```python
from build123d import *

# Parameters (mm, degrees)
EXTRUDE004_DEPTH                     = 120
EXTRUDE004_ONTO_SKETCH004_ROLL_ANGLE = 90
ARRAY005_X_COUNT                     = 2
ARRAY005_X_PITCH                     = 51
EXTRUDE001_DEPTH                     = 120
EXTRUDE001_ONTO_SKETCH001_ROLL_ANGLE = 90
ARRAY003_Z_COUNT                     = 2
ARRAY003_Z_PITCH                     = 21
BOX001_W                             = 96
BOX001_H                             = 118
BOX001_DEPTH                         = 41
BOX_W                                = 102
BOX_H                                = 120
BOX_DEPTH                            = 47
FILLET_R                             = 0.5
EXTRUDE003_DEPTH                     = 119
EXTRUDE003_ONTO_SKETCH003_ROLL_ANGLE = 90
ARRAY_X_COUNT                        = 2
ARRAY_X_PITCH                        = 51
EXTRUDE002_DEPTH                     = 119
EXTRUDE002_ONTO_SKETCH002_ROLL_ANGLE = 90
ARRAY004_Z_COUNT                     = 2
ARRAY004_Z_PITCH                     = 21
EXTRUDE_DEPTH                        = 0.8
ARRAY002_X_COUNT                     = 8
ARRAY002_X_PITCH                     = 12


with BuildPart() as bottomsideguidearray:
    # Sketch004 as drawn → Extrude004 (new)
    with BuildSketch(Plane.XY):
        Polygon((-6, 1), (4, 1), (2, -1), (-4, -1), align=None)
    extrude(amount=-EXTRUDE004_DEPTH)


with BuildPart() as bottomsideguidearray_1:
    # Extrude004 onto Sketch004 roll: moved
    add(bottomsideguidearray.part.rotate(Axis((0, 0, 0), (1, 0, 0)), EXTRUDE004_ONTO_SKETCH004_ROLL_ANGLE))


with BuildPart() as bottomsideguidearray_2:
    # Extrude004 onto Sketch004 placement: moved
    add(bottomsideguidearray_1.part)


with BuildPart() as bottomsideguidearray_3:
    # Extrude004 placement: moved
    add(bottomsideguidearray_2.part.moved(Location((25.5, 0, 0))))

    # Array005 X: BottomSideGuideArray ×2


with BuildPart() as bottomsideguidearray_4:
    add(bottomsideguidearray_3.part)
    with Locations(*[(i * ARRAY005_X_PITCH, 0, 0) for i in range(1, ARRAY005_X_COUNT)]):
        add(bottomsideguidearray_3.part)


with BuildPart() as guidegaps:
    # Sketch001 as drawn → Extrude001 (new)
    with BuildSketch(Plane.XY):
        Polygon((0, 0), (0, 10), (2, 8), (2, 2), align=None)
    extrude(amount=-EXTRUDE001_DEPTH)


with BuildPart() as guidegaps_1:
    # Extrude001 onto Sketch001 roll: moved
    add(guidegaps.part.rotate(Axis((0, 0, 0), (1, 0, 0)), EXTRUDE001_ONTO_SKETCH001_ROLL_ANGLE))


with BuildPart() as guidegaps_2:
    # Extrude001 onto Sketch001 placement: moved
    add(guidegaps_1.part.moved(Location((99, 0, 7))))

    # Array003 Z: GuideGaps ×2


with BuildPart() as guidegaps_3:
    add(guidegaps_2.part)
    with Locations(*[(0, 0, i * ARRAY003_Z_PITCH) for i in range(1, ARRAY003_Z_COUNT)]):
        add(guidegaps_2.part)

    # Fusion003: union BottomSideGuideArray
    add(bottomsideguidearray_4.part)


with BuildPart() as inner_box:
    # Box001 → Box001 (new body)
    with BuildSketch(Plane(origin=(2, 0, 2), x_dir=(1, 0, 0), z_dir=(0, 0, 1))):
        with Locations((48, 59)):
            Rectangle(BOX001_W, BOX001_H)
    extrude(amount=BOX001_DEPTH)


with BuildPart() as filletedcase:
    # Box → Box (new body)
    with BuildSketch(Plane(origin=(-1, 0, -1), x_dir=(1, 0, 0), z_dir=(0, 0, 1))):
        with Locations((51, 60)):
            Rectangle(BOX_W, BOX_H)
    extrude(amount=BOX_DEPTH)

    # Cut: cut Inner Box
    add(inner_box.part, mode=Mode.SUBTRACT)

    # Fillet
    fillet_edges = [filletedcase.edges().sort_by_distance(p)[0] for p in [
        (-1, 0, 22.5),
        (-1, 60, 46),
        (-1, 120, 22.5),
        (-1, 60, -1),
        (50, 0, -1),
        (101, 0, 22.5),
        (50, 0, 46),
        (50, 120, 46),
        (101, 60, 46),
        (50, 120, -1),
        (101, 120, 22.5),
        (101, 60, -1),
    ]]
    fillet(fillet_edges, radius=FILLET_R)


with BuildPart() as topsideguidearray:
    # Sketch003 as drawn → Extrude003 (new)
    with BuildSketch(Plane.XY):
        Polygon((-5.2, 47.6), (3.2, 47.6), (1.6, 46), (-3.6, 46), align=None)
    extrude(amount=-EXTRUDE003_DEPTH)


with BuildPart() as topsideguidearray_1:
    # Extrude003 onto Sketch003 roll: moved
    add(topsideguidearray.part.rotate(Axis((0, 0, 0), (1, 0, 0)), EXTRUDE003_ONTO_SKETCH003_ROLL_ANGLE))


with BuildPart() as topsideguidearray_2:
    # Extrude003 onto Sketch003 placement: moved
    add(topsideguidearray_1.part)


with BuildPart() as topsideguidearray_3:
    # Extrude003 placement: moved
    add(topsideguidearray_2.part.moved(Location((25.5, 1, 0))))

    # Array X: TopSideGuideArray ×2


with BuildPart() as topsideguidearray_4:
    add(topsideguidearray_3.part)
    with Locations(*[(i * ARRAY_X_PITCH, 0, 0) for i in range(1, ARRAY_X_COUNT)]):
        add(topsideguidearray_3.part)


with BuildPart() as guiderods:
    # Sketch002 as drawn → Extrude002 (new)
    with BuildSketch(Plane.XY):
        Polygon((0.4, 9.2), (0.4, 0.8), (2, 2.4), (2, 7.6), align=None)
    extrude(amount=-EXTRUDE002_DEPTH)


with BuildPart() as guiderods_1:
    # Extrude002 onto Sketch002 roll: moved
    add(guiderods.part.rotate(Axis((0, 0, 0), (1, 0, 0)), EXTRUDE002_ONTO_SKETCH002_ROLL_ANGLE))


with BuildPart() as guiderods_2:
    # Extrude002 onto Sketch002 placement: moved
    add(guiderods_1.part.moved(Location((-1, 0, 7))))


with BuildPart() as guiderods_3:
    # Extrude002 placement: moved
    add(guiderods_2.part.moved(Location((-2, 1, 0))))

    # Array004 Z: GuideRods ×2


with BuildPart() as guiderods_4:
    add(guiderods_3.part)
    with Locations(*[(0, 0, i * ARRAY004_Z_PITCH) for i in range(1, ARRAY004_Z_COUNT)]):
        add(guiderods_3.part)

    # Fusion002: union TopSideGuideArray
    add(topsideguidearray_4.part)


with BuildPart() as finalcabinet:
    # Sketch → Extrude (new body)
    with BuildSketch(Plane.XY):
        Polygon((0.5, 0), (0.25, 104), (0.25, 105), (1.75, 105), (1.75, 104), (1.5, 0), align=None)
    extrude(amount=EXTRUDE_DEPTH)

    # Array002 X: FinalCabinet ×8


with BuildPart() as finalcabinet_1:
    add(finalcabinet.part)
    with Locations(*[(i * ARRAY002_X_PITCH, 0, 0) for i in range(1, ARRAY002_X_COUNT)]):
        add(finalcabinet.part)


with BuildPart() as finalcabinet_2:
    # Array002 placement: moved
    add(finalcabinet_1.part.moved(Location((7, 13, 2))))

    # Fusion: union FilletedCase, GuideRods
    add(filletedcase.part)
    add(guiderods_4.part)

    # Cut001: cut GuideGaps
    add(guidegaps_3.part, mode=Mode.SUBTRACT)


solid = finalcabinet_2.part
```
Verification items for the finished model (mm, model axes). A direction names the side the tool comes from. Round coordinates to 2 decimals unless told otherwise and drop trailing zeros. Write each loop counter-clockwise with the first axis right and the second up, starting at its lowest first coordinate (ties: lowest second). Pieces come first, ordered by that corner, then holes.
1. Scan lines: L1, parallel to Z at x = 26, y = 96; L2, parallel to X at y = 102, z = 32; L3, parallel to Z at x = 37, y = 70. Record each from-to range of solid material in increasing order.
2. Section check B-B on z = 23.5. Enter the section's corners in (x, y), plus the area to 3 significant figures.
3. Section check A-A on x = 76. Enter the section's corners in (y, z).
4. Access from +Z, -Z, +X, -X, +Y, -Y to the whole of each face (thin tool, end or side, straight path). Record for faces 1 (the flat face through (2, 58, 22)), 2 (the flat face through (99, 59, 12)), 3 (the flat face through (10, 61, -1)).
5. Draft check along Z on faces 4 (the flat face through (50, 0, 0)), 5 (the flat face through (99, 59, 33)), 6 (the flat face through (24, 60, 47.6)), 7 (the flat face through (98, 58, 22)). Enter one of: +Z half, -Z half, draft (parallel to the pull), parting line (faces both ways), or undercut.
6. Gauge pin test, flat ends, axial feed: P1, Ø0.6, axis at y = 117.5, z = 2.5, coming from the -X side; P2, Ø1.2, axis at x = 8, y = 52, coming from the +Z side; P3, Ø1.5, axis at x = 82.5, z = 5.5, coming from the -Y side. Record the tip position at first contact, or that the pin passes through.
7. Section check C-C on x = 64. Enter the section's corners in (y, z).
Answer:
1. L1: z = 1 to 2, 43 to 47.6
1. L2: x = -2.6 to 2, 98 to 99
1. L3: z = -1 to 2, 43 to 46
2. outline: (-1, 0.5) arc R0.5 ccw to (-0.5, 0) - (2, 0) - (2, 118) - (98, 118) - (98, 0) - (100.5, 0) arc R0.5 ccw to (101, 0.5) - (101, 119.5) arc R0.5 ccw to (100.5, 120) - (-0.5, 120) arc R0.5 ccw to (-1, 119.5) - close
2. area: 912 mm2
3. outline: (0, 1) - (120, 1) - (120, 45.5) arc R0.5 ccw to (119.5, 46) - (120, 46) - (120, 47.6) - (1, 47.6) - (1, 46) - (0.5, 46) arc R0.5 ccw to (0, 45.5) - (0, 43) - (118, 43) - (118, 2) - (0, 2) - close
4. face 1: -Y
4. face 2: +Y, -Y
4. face 3: -Z, +X, -X, +Y, -Y
5. face 4: draft
5. face 5: undercut
5. face 6: +Z half
5. face 7: undercut
6. P1: stops at x = -1
6. P2: stops at z = 46
6. P3: stops at y = 118
7. outline: (0, -0.5) arc R0.5 ccw to (0.5, -1) - (119.5, -1) arc R0.5 ccw to (120, -0.5) - (120, 45.5) arc R0.5 ccw to (119.5, 46) - (0.5, 46) arc R0.5 ccw to (0, 45.5) - (0, 43) - (118, 43) - (118, 2) - (0, 2) - close
